Work out the finished part from the listing and answer in its coordinate system (mm). Face numbers are marked on the shaded views. A direction names the side the tool comes from. Coordinates: 2 decimals unless noted, no trailing zeros. Order: outer loops, then holes, each group sorted by start corner. A loop starts at its lowest first (then second) coordinate and runs counter-clockwise, first axis right, second up. Notation, with made-up numbers: M -14.75,82 L 40.25,82 A33 cw 40.25,113 Z; hole C -2,45 d7. An arc over 180 degrees is marked long. Use a Markdown table: item, result.
from build123d import *

# Parameters (mm, degrees)
F0_W     = 11.7570459843
F0_H     = 83.8521160185
F0_W_2   = 109.5845103264
F0_W_3   = 29.9471821636
F0_H_2   = 36.8239460513
F1_DEPTH = 2
F2_DEPTH = 10
F3_DEPTH = 20


with BuildPart() as f1:
    # F0 (on Top) → F1 (new body)
    with BuildSketch(Plane.XY):
        with Locations((58.1197217107, -1.4419015497)):
            Rectangle(F0_W, F0_H)
        with Locations((-2.5510564446, -1.4419015497)):
            Rectangle(F0_W_2, F0_H)
        with Locations((-35.9366210178, 6.5440149046)):
            Rectangle(F0_W_3, F0_H_2, mode=Mode.SUBTRACT)
        with Locations((-35.9366210178, 6.5440149046)):
            Rectangle(F0_W_3, F0_H_2)
    extrude(amount=-F1_DEPTH)

    # F0 (on Top) → F2 (join)
    with BuildSketch(Plane.XY):
        with Locations((-35.9366210178, 6.5440149046)):
            Rectangle(F0_W_3, F0_H_2)
    extrude(amount=F2_DEPTH)

    # F0 (on Top) → F3 (join)
    with BuildSketch(Plane.XY):
        with Locations((58.1197217107, -1.4419015497)):
            Rectangle(F0_W, F0_H)
    extrude(amount=F3_DEPTH)


solid = f1.part
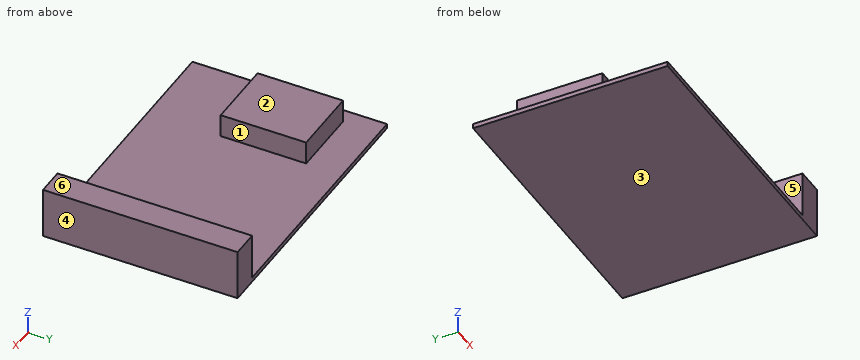
(1) Straight lines are drawn through the part: L1, parallel to X at y = 11.5, z = 9.75; L2, parallel to Z at x = 26.5, y = 3; L3, parallel to Z at x = -26, y = -9.5. For each, find the intervals that lie inside material, in ascending order.
Conclusion:
| item | result |
|---|---|
| L1 | -50.91 to -20.96, 52.24 to 64 |
| L2 | -2 to 0 |
| L3 | -2 to 10 |
(2) A cutting plane is placed at A-A (z = 5). Determine the outline of the cut face in (x, y), then the cut area to 3 significant figures.
Conclusion:
| item | result |
|---|---|
| outline | M -50.91,-11.87 L -20.96,-11.87 L -20.96,24.96 L -50.91,24.96 Z; M 52.24,-43.37 L 64,-43.37 L 64,40.48 L 52.24,40.48 Z |
| area | 2,090 mm2 |
(3) Given P1, Ø5, axis at x = -33.5, z = 4, coming from the +Y side; P2, Ø5, axis at y = 11.5, z = 4, coming from the -X side; P3, Ø15, axis at x = -36, y = 7, coming from the +Z side, each flat-ended and moving along its own axis, determine where each tip first touches the part or whether it passes through.
Conclusion:
| item | result |
|---|---|
| P1 | y = 24.96 |
| P2 | x = -50.91 |
| P3 | z = 10 |
(4) A cutting plane is placed at C-C (x = -15). Determine the outline of the cut face in (y, z).
Conclusion:
| item | result |
|---|---|
| outline | M -43.37,-2 L 40.48,-2 L 40.48,0 L -43.37,0 Z |
(5) A cutting plane is placed at D-D (z = 12.75). Determine the outline of the cut face in (x, y).
Conclusion:
| item | result |
|---|---|
| outline | M 52.24,-43.37 L 64,-43.37 L 64,40.48 L 52.24,40.48 Z |
(6) Determine the mould class of the marked faces 4, 5 and 6 for opening direction X: pulls with the +X half, pulls with the -X half, needs draft (parallel to the pull), parting line crosses it, or undercut.
Conclusion:
| item | result |
|---|---|
| face 4 | pulls with the +X half |
| face 5 | undercut |
| face 6 | needs draft |
(7) Which of the six approach directions +Z, -Z, +X, -X, +Y, -Y give full straight-line access (tool end or side, diameter ignored) to the marked faces 1, 2 and 3?
Conclusion:
| item | result |
|---|---|
| face 1 | +Z, +Y, -Y |
| face 2 | +Z, -X, +Y, -Y |
| face 3 | -Z, +X, -X, +Y, -Y |
(8) A cutting plane is placed at B-B (y = 13). Determine the outline of the cut face in (x, z), then the cut area to 3 significant figures.
Conclusion:
| item | result |
|---|---|
| outline | M -57.34,-2 L 64,-2 L 64,20 L 52.24,20 L 52.24,0 L -20.96,0 L -20.96,10 L -50.91,10 L -50.91,0 L -57.34,0 Z |
| area | 777 mm2 |
